For this review, take the finished solid that the model builds, in its own axes (mm). Face numbers are marked on the shaded views. A direction names the side the tool comes from. Give positions to 0.01 mm unless a question says otherwise; leave off trailing zeros. Write each loop counter-clockwise with the first axis right and the second up, starting at its lowest first coordinate (ties: lowest second). Pieces come first, ordered by that corner, then holes. Notation, with made-up numbers: M -5.75,3 L 47.25,3 A19 cw 47.25,14 Z; hole C -6.75,68 d8. An arc over 180 degrees is marked long. One line per item, written item: value. Start each with the question number.
Item 1: Consider section B-B, the plane z = -44.75. Write out the cut boundary in (x, y).
Item 2: Consider section C-C, the plane x = -27.5. Write out the cut boundary in (y, z), and give its area (3 significant figures).
Item 3: Clearance check with flat-ended pins moving along their axes: pin 1 Ø4 at (x, z) = (-22, -44.5) entering from +Y; pin 2 Ø1.5 at (y, z) = (8, -47) entering from -X; pin 3 Ø1.5 at (x, y) = (-24, 3) entering from -Z. State where each tip first meets the part, or that it passes through.
Item 4: Tool access review of the marked faces 4, 5, 6, 7 and 8: name each direction out of +Z, -Z, +X, -X, +Y, -Y from which nothing blocks a thin tool from reaching the whole face with its end or side.
Item 5: Mouldability with a two-part tool opening along X and no side actions: class the marked faces 1, 2 and 3 as released by +X, released by -X, zero draft, split by the parting line, or undercut.
Item 6: To check wall thickness, follow probe 1 along Z at (x, y) = (-25.75, 5); probe 2 along Z at (x, y) = (-20.5, 9.75); probe 3 along X at (y, z) = (7.25, -40.25). State the ranges of each line that lie inside material, in increasing order.
Item 7: Consider section A-A, the plane y = 6.5. Write out the cut boundary in (x, z).
Item 8: Consider section D-D, the plane x = -29.5. Write out the cut boundary in (y, z).
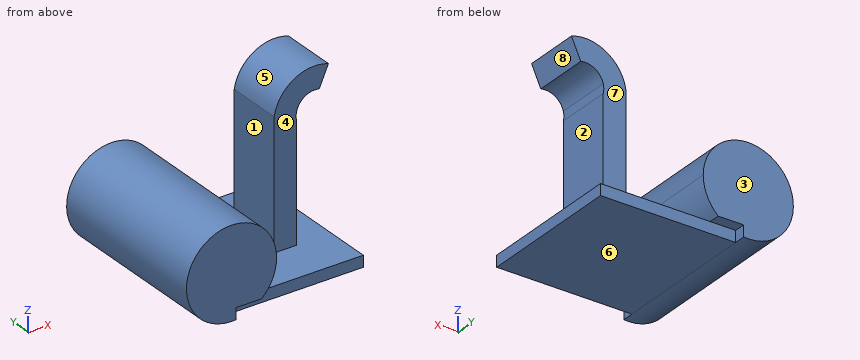
```python
from build123d import *

# Parameters (mm, degrees)
BOSS_EXTRUDE1_DEPTH = 15
SKETCH2_W           = 12
SKETCH2_H           = 1
CUT_EXTRUDE1_DEPTH  = 1
SKETCH5_W           = 6.028776927
SKETCH5_H           = 6.351314433
SKETCH5_W_2         = 5.976909526
SKETCH5_H_2         = 6.219071559
CUT_EXTRUDE2_DEPTH  = 21


with BuildPart() as part:
    # Sketch1 → Boss-Extrude1 (new body)
    with BuildSketch(Plane(origin=(0, 0, 0), x_dir=(1, 0, 0), z_dir=(0, 1, 0))):
        with BuildLine():
            ThreePointArc((-26.508767977, 45.209827562), (-26.856482836, 46.841027505), (-27.839174603, 48.188631218))
            Line((-27.839174603, 48.188631218), (-30.097524166, 48.188631218))
            Line((-30.097524166, 48.188631218), (-30.097524166, 49.188631218))
            ThreePointArc((-30.097524166, 49.188631218), (-33.479035241, 42.530739587), (-26.508767977, 45.209827562))
        make_face()
        with BuildLine():
            Line((-30.097524166, 48.188631218), (-27.839174603, 48.188631218))
            ThreePointArc((-27.839174603, 48.188631218), (-28.889234266, 48.86730081), (-30.097524166, 49.188631218))
            Line((-30.097524166, 49.188631218), (-30.097524166, 48.188631218))
        make_face()
        with BuildLine():
            Line((-27.839174603, 48.188631218), (-23.179530848, 48.188631218))
            Line((-23.179530848, 48.188631218), (-21.179530848, 48.188631218))
            Line((-21.179530848, 48.188631218), (-18.097524166, 48.188631218))
            Line((-18.097524166, 48.188631218), (-18.097524166, 49.188631218))
            Line((-18.097524166, 49.188631218), (-30.097524166, 49.188631218))
            ThreePointArc((-30.097524166, 49.188631218), (-28.889234266, 48.86730081), (-27.839174603, 48.188631218))
        make_face()
        with BuildLine():
            Line((-23.179530848, 48.188631218), (-23.179530848, 38.073593242))
            ThreePointArc((-23.179530848, 38.073593242), (-22.504394786, 39.656834499), (-21.179530848, 40.755559728))
            Line((-21.179530848, 40.755559728), (-21.179530848, 48.188631218))
            Line((-21.179530848, 48.188631218), (-23.179530848, 48.188631218))
        make_face()
        with BuildLine():
            Line((-21.179530848, 36.869987329), (-21.179530848, 37.062229248))
            ThreePointArc((-21.179530848, 37.062229248), (-21.23095476, 37.471790285), (-21.179530848, 37.881351323))
            Line((-21.179530848, 37.881351323), (-21.179530848, 40.755559728))
            ThreePointArc((-21.179530848, 40.755559728), (-22.504394786, 39.656834499), (-23.179530848, 38.073593242))
            Line((-23.179530848, 38.073593242), (-23.179530848, 36.869987329))
            Line((-23.179530848, 36.869987329), (-21.179530848, 36.869987329))
        make_face()
        with BuildLine():
            Line((-18.360117838, 34.024219809), (-19.183298893, 35.861921993))
            ThreePointArc((-19.183298893, 35.861921993), (-20.42797821, 36.052015934), (-21.179530848, 37.062229248))
            Line((-21.179530848, 37.062229248), (-21.179530848, 36.869987329))
            Line((-21.179530848, 36.869987329), (-23.179530848, 36.869987329))
            ThreePointArc((-23.179530848, 36.869987329), (-21.43275623, 34.324403792), (-18.360117838, 34.024219809))
        make_face()
    extrude(amount=BOSS_EXTRUDE1_DEPTH)

    # Sketch2 → Cut-Extrude1 (cut)
    with BuildSketch(Plane(origin=(0, 0, -49.188631218), x_dir=(-1, 0, 0), z_dir=(0, 0, -1))):
        with Locations((24.097524166, 14.5)):
            Rectangle(SKETCH2_W, SKETCH2_H)
        with Locations((24.097524166, 0.5)):
            Rectangle(SKETCH2_W, SKETCH2_H)
    extrude(amount=-CUT_EXTRUDE1_DEPTH, mode=Mode.SUBTRACT)

    # Sketch5 → Cut-Extrude2 (cut)
    with BuildSketch(Plane(origin=(0, 0, -48.188631218), x_dir=(-1, 0, 0), z_dir=(0, 0, -1))):
        with Locations((20.800096239, 13.175657217)):
            Rectangle(SKETCH5_W, SKETCH5_H)
        with Locations((20.774162538, 1.89046422)):
            Rectangle(SKETCH5_W_2, SKETCH5_H_2)
    extrude(amount=-CUT_EXTRUDE2_DEPTH, mode=Mode.SUBTRACT)


solid = part.part
```
Model answer:
1. outline: M -34.48,0 L -26.54,0 L -26.54,15 L -34.48,15 Z; M -23.18,5 L -21.18,5 L -21.18,10 L -23.18,10 Z
2. outline: M 0,-47.85 L 15,-47.85 L 15,-42.57 L 0,-42.57 Z; M 1,-49.19 L 14,-49.19 L 14,-48.19 L 1,-48.19 Z
2. area: 92.1 mm2
3. pin 1: stops at y = 10
3. pin 2: stops at x = -34.37
3. pin 3: stops at z = -49.19
4. face 4: +Z, +X, -Y
4. face 5: +Z, +Y, -Y
4. face 6: -Z, +X, +Y, -Y
4. face 7: +Z, +X, +Y
4. face 8: +X, +Y, -Y
5. face 1: undercut
5. face 2: released by +X
5. face 3: zero draft
6. probe 1: z = -49.19 to -48.19
6. probe 2: z = -49.19 to -48.19, -36.1 to -33.94
6. probe 3: x = -23.18 to -21.18
7. outline: M -30.1,-49.19 L -18.1,-49.19 L -18.1,-48.19 L -21.18,-48.19 L -21.18,-37.88 A1.66 cw -19.18,-35.86 L -18.36,-34.02 A3.66 ccw -23.18,-36.87 L -23.18,-48.19 L -27.84,-48.19 A4 ccw long Z
8. outline: M 0,-48.19 L 1,-48.19 L 1,-49.19 L 14,-49.19 L 14,-48.19 L 15,-48.19 L 15,-41.34 L 0,-41.34 Z
